Input: part model. Units: mm. Frame: model coordinates. A direction names the side the tool comes from. Give positions to 0.01 mm unless a question says otherwise; leave off trailing zeros. Loops run counter-clockwise (first coordinate to the right, second up) from the corner with the lowest first, then second, coordinate; pieces in that order, holes last. Notation, with made-up numbers: (36.25, 3.5) - (85.25, 3.5) arc R29 cw to (85.25, 33.5) - close; hole circle Ø4 at (13, 8). An arc over 180 degrees is marked (long way). One line per question, with ' | ' between items. Start each with the question number.
from build123d import *

# Parameters (mm, degrees)
PAD_DEPTH       = 12
FILLET_R        = 1
FILLET001_R     = 1
FILLET002_R     = 1
FILLET003_R     = 1
POCKET_DEPTH    = 5
PAD001_DEPTH    = 4
SKETCH004_R     = 2.25
PAD002_DEPTH    = 3
POCKET001_DEPTH = 5


with BuildPart() as part:
    # Sketch → Pad (new body)
    with BuildSketch(Plane.XY):
        Polygon((-15.25744, 12.972063), (7.84256, 12.972063), (7.84256, 8.272063), (12.49256, 8.272063), (12.49256, 5.972063), (7.84256, 5.972063), (7.84256, -10.127937), (-15.25744, -10.127937), (-15.25744, 5.972063), (-19.90744, 5.972063), (-19.90744, 8.272063), (-15.25744, 8.272063), align=None)
    extrude(amount=PAD_DEPTH)

    # Fillet
    fillet_edges = [part.edges().sort_by_distance(p)[0] for p in [
        (-15.25744, -2.077937, 12),
    ]]
    fillet(fillet_edges, radius=FILLET_R)

    # Fillet001
    fillet001_edges = [part.edges().sort_by_distance(p)[0] for p in [
        (-15.25744, -2.077937, 0),
    ]]
    fillet(fillet001_edges, radius=FILLET001_R)

    # Fillet002
    fillet002_edges = [part.edges().sort_by_distance(p)[0] for p in [
        (7.84256, -2.077937, 0),
    ]]
    fillet(fillet002_edges, radius=FILLET002_R)

    # Fillet003
    fillet003_edges = [part.edges().sort_by_distance(p)[0] for p in [
        (7.84256, -2.077937, 12),
    ]]
    fillet(fillet003_edges, radius=FILLET003_R)

    # Sketch001 → Pocket (cut)
    with BuildSketch(Plane(origin=(0, 8.272063, 0), x_dir=(-1, 0, 0), z_dir=(0, 1, 0))):
        with BuildLine():
            ThreePointArc((-11.368116, 5.5), (-8.868116, 6), (-11.368116, 6.5))
            Line((-12.49256, 6.5), (-11.368116, 6.5))
            Line((-12.49256, 5.5), (-12.49256, 6.5))
            Line((-11.368116, 5.5), (-12.49256, 5.5))
        make_face()
    extrude(amount=-POCKET_DEPTH, mode=Mode.SUBTRACT)

    # Sketch003 → Pad001 (new body)
    with BuildSketch(Plane(origin=(0, 12.972063, 0), x_dir=(-1, 0, 0), z_dir=(0, 1, 0))):
        with BuildLine():
            ThreePointArc((3.52244, 8.068641), (-7.59256, 6), (3.52244, 3.931359))
            ThreePointArc((3.52244, 3.931359), (6.65744, 6), (3.52244, 8.068641))
        make_face()
    extrude(amount=PAD001_DEPTH)

    # Sketch004 → Pad002 (new body)
    with BuildSketch(Plane(origin=(0, 16.972063, 0), x_dir=(-1, 0, 0), z_dir=(0, 1, 0))):
        with Locations((-1.84256, 6)):
            Circle(SKETCH004_R)
    extrude(amount=PAD002_DEPTH)

    # Sketch005 → Pocket001 (cut)
    with BuildSketch(Plane(origin=(0, 8.272063, 0), x_dir=(-1, 0, 0), z_dir=(0, 1, 0))):
        with BuildLine():
            ThreePointArc((18.643443, 6.5), (16.143443, 6), (18.643443, 5.5))
            Line((19.90744, 5.5), (18.643443, 5.5))
            Line((19.90744, 6.5), (19.90744, 5.5))
            Line((18.643443, 6.5), (19.90744, 6.5))
        make_face()
    extrude(amount=-POCKET001_DEPTH, mode=Mode.SUBTRACT)


solid = part.part
Q1. Section B-B, the plane z = 6. Output: boundary loops of the cut face in (x, y), plus the area to 3 significant figures.
Q2. First-contact query: pin 1 (4.5 mm diameter, centred on x = 11, z = 7, fed in from -Y); pin 2 (2.5 mm diameter, centred on x = 10.17, z = 6, fed in from +Y); pin 3 (5 mm diameter, centred on y = -4, z = 5.5, fed in from -X); pin 4 (1.4 mm diameter, centred on y = 11, z = 4, fed in from +X). Flat tips, straight axial feed; report the tip coordinate or a pass-through.
Q3. Access query for faces 1 (the face through (-15.257, 11, 6)), 2 (the face through (-19, 7, 5.5)), 3 (the face through (7.557, -2.191, 0.301)), 4 (the face through (9.6, 8.272, 4.6)). Directions: +Z, -Z, +X, -X, +Y, -Y. A direction counts if a zero-diameter tool reaches every point of the face in a straight line with its end or side. Return the directions, or none.
Q4. Section C-C, the plane y = -3. Output: boundary loops of the cut face in (x, z), plus the area to 3 significant figures.
Q5. Section A-A, the plane x = 10.5. Output: boundary loops of the cut face in (y, z), plus the area to 3 significant figures.
Q6. Draft query along X for faces 5 (the face through (-19, 7, 6.5)), 6 (the face through (-14.97, -1.97, 11.7)), 7 (the face through (-16.144, 7.138, 6.05)). Return one class per face: +X half, -X half, draft (parallel to the pull), parting line (faces both ways), or undercut.
Q7. Section D-D, the plane x = 3.5. Output: boundary loops of the cut face in (y, z).
Q8. Line query: L1, parallel to Y at x = -11.5, z = 8.25; L2, parallel to X at y = 0, z = 10.75; L3, parallel to X at y = 7, z = 6.75. Output: solid intervals per line, ascending. Write a range as from..to.
Solved:
1) outline: (-16.14, 5.97) - (-15.26, 5.97) - (-15.26, -10.13) - (7.84, -10.13) - (7.84, 5.97) - (8.87, 5.97) - (8.87, 8.27) - (7.84, 8.27) - (7.84, 12.97) - (7.59, 12.97) - (7.59, 16.97) - (4.09, 16.97) - (4.09, 19.97) - (-0.41, 19.97) - (-0.41, 16.97) - (-6.66, 16.97) - (-6.66, 12.97) - (-15.26, 12.97) - (-15.26, 8.27) - (-16.14, 8.27) - close | area: 609 mm²
2) pin 1: stops at y = 5.97 | pin 2: passes through | pin 3: stops at x = -15.26 | pin 4: stops at x = 7.84
3) face 1: +Z, -Z, -X, +Y | face 2: -X, +Y, -Y | face 3: -Z, +X, -Y | face 4: +Z, -Z, +X, +Y
4) outline: (-15.26, 1) arc R1 ccw to (-14.26, 0) - (6.84, 0) arc R1 ccw to (7.84, 1) - (7.84, 11) arc R1 ccw to (6.84, 12) - (-14.26, 12) arc R1 ccw to (-15.26, 11) - close | area: 276 mm²
5) outline: (5.97, 0) - (8.27, 0) - (8.27, 4.74) - (5.97, 4.74) - close; (5.97, 7.26) - (8.27, 7.26) - (8.27, 12) - (5.97, 12) - close | area: 21.8 mm²
6) face 5: draft | face 6: -X half | face 7: undercut
7) outline: (-10.13, 0) - (12.97, 0) - (12.97, 0.49) - (16.97, 0.49) - (16.97, 4.48) - (19.97, 4.48) - (19.97, 7.52) - (16.97, 7.52) - (16.97, 11.51) - (12.97, 11.51) - (12.97, 12) - (-10.13, 12) - close
8) L1: y = -10.13..12.97 | L2: x = -15.26..7.84 | L3: x = -19.91..-18.51, -16.38..9.11, 11.23..12.49
